Design review of the part built by this model. Coordinates are the model's own, in mm. Give positions to 0.01 mm unless a question says otherwise; leave off trailing zeros. Loops run counter-clockwise (first coordinate to the right, second up) from the corner with the lowest first, then second, coordinate; pieces in that order, holes last. Notation, with made-up numbers: (-4.5, 40) -> (45.5, 40) arc R24 cw to (45.5, 66) -> close; hole circle Ø4 at (73.5, 76). An arc over 180 degrees is marked (long way). Answer in a Markdown table with one row per item. Add a question column.
(1) For line 1 (Y direction, x = -35, z = 2.15); line 2 (X direction, y = -26.5, z = 2.3); line 3 (Y direction, x = -70.5, z = 1.65), list the stretches that pass through material, from the lowest coordinate up.
(2) Consider section A-A on y = -7.5. Write out the cut boundary in (x, z).
(3) For pin 1 (1.5 mm diameter, centred on x = -62, y = -69, fed in from +Z) (3 decimals), flat-tipped, find the tip position at first contact; note if it passes through.
(4) Consider section C-C on y = -75. Write out the cut boundary in (x, z).
(5) Consider section D-D on x = -2.5. Write out the cut boundary in (y, z), then the cut area to 3 significant figures.
(6) Consider section B-B on x = -71.5. Write out the cut boundary in (y, z).
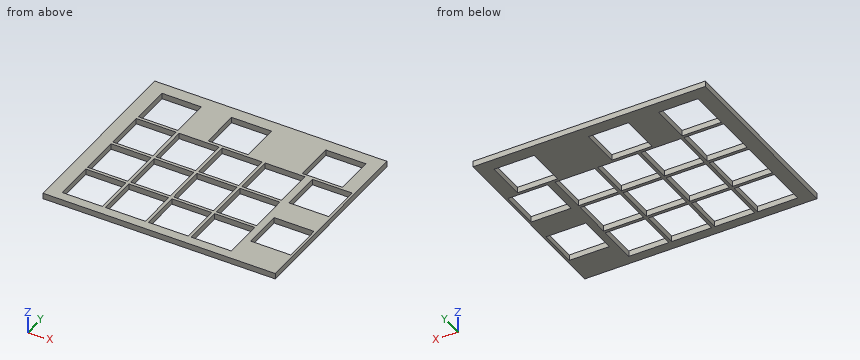
from build123d import *

# Parameters (mm, degrees)
F0_W      = 100
F0_H      = 82
F1_DEPTH  = 2.5
F2_W      = 17.2
F2_H      = 17.2
F3_DEPTH  = 25
F2_W_2    = 17.030713
F4_DEPTH  = 25
F5_W      = 17.2
F5_H      = 17.2
F6_DEPTH  = 25
F7_W      = 17.2
F7_H      = 17.2
F8_DEPTH  = 25
F9_W      = 17.2
F9_H      = 17.2
F10_DEPTH = 25
F11_W     = 17.2
F11_H     = 17.2
F12_DEPTH = 25
F13_W     = 17.2
F13_H     = 17.2
F14_DEPTH = 25
F15_W     = 17.2
F15_H     = 17.2
F16_DEPTH = 25


with BuildPart() as f1:
    # F0 (on Top) → F1 (new body)
    with BuildSketch(Plane.XY):
        with Locations((-39.136762, -41)):
            Rectangle(F0_W, F0_H)
    extrude(amount=F1_DEPTH)

    # F2 (on face) → F3 (cut)
    with BuildSketch(Plane.XY.offset(2.5)):
        with Locations((-74.536762, -69.4)):
            Rectangle(F2_W, F2_H)
    extrude(amount=-F3_DEPTH, mode=Mode.SUBTRACT)

    # F2 (on face) → F4 (cut)
    with BuildSketch(Plane.XY.offset(2.5)):
        with Locations((-74.536762, -69.4)):
            Rectangle(F2_W, F2_H)
        with Locations((-74.536762, -50.9)):
            Rectangle(F2_W, F2_H)
        with Locations((-74.536762, -32.4)):
            Rectangle(F2_W, F2_H)
        with Locations((-74.452118, -13.9)):
            Rectangle(F2_W_2, F2_H)
    extrude(amount=-F4_DEPTH, mode=Mode.SUBTRACT)

    # F5 (on face) → F6 (cut)
    with BuildSketch(Plane.XY.offset(2.5)):
        with Locations((-56.036762, -69.4)):
            Rectangle(F5_W, F5_H)
        with Locations((-37.536762, -69.4)):
            Rectangle(F5_W, F5_H)
        with Locations((-19.036762, -69.4)):
            Rectangle(F5_W, F5_H)
    extrude(amount=-F6_DEPTH, mode=Mode.SUBTRACT)

    # F7 (on face) → F8 (cut)
    with BuildSketch(Plane.XY.offset(2.5)):
        with Locations((-56.036762, -50.9)):
            Rectangle(F7_W, F7_H)
        with Locations((-56.036762, -32.4)):
            Rectangle(F7_W, F7_H)
        with Locations((-37.536762, -50.9)):
            Rectangle(F7_W, F7_H)
        with Locations((-37.536762, -32.4)):
            Rectangle(F7_W, F7_H)
    extrude(amount=-F8_DEPTH, mode=Mode.SUBTRACT)

    # F9 (on face) → F10 (cut)
    with BuildSketch(Plane.XY.offset(2.5)):
        with Locations((-19.036762, -50.9)):
            Rectangle(F9_W, F9_H)
        with Locations((-19.036762, -32.4)):
            Rectangle(F9_W, F9_H)
    extrude(amount=-F10_DEPTH, mode=Mode.SUBTRACT)

    # F11 (on face) → F12 (cut)
    with BuildSketch(Plane.XY.offset(2.5)):
        with Locations((1.263238, -60.4)):
            Rectangle(F11_W, F11_H)
        with Locations((1.263238, -32.4)):
            Rectangle(F11_W, F11_H)
    extrude(amount=-F12_DEPTH, mode=Mode.SUBTRACT)

    # F13 (on face) → F14 (cut)
    with BuildSketch(Plane.XY.offset(2.5)):
        with Locations((-44.336762, -13.9)):
            Rectangle(F13_W, F13_H)
    extrude(amount=-F14_DEPTH, mode=Mode.SUBTRACT)

    # F15 (on face) → F16 (cut)
    with BuildSketch(Plane.XY.offset(2.5)):
        with Locations((-3.736762, -13.9)):
            Rectangle(F15_W, F15_H)
    extrude(amount=-F16_DEPTH, mode=Mode.SUBTRACT)


solid = f1.part
Values follow:
| question | item | result |
|---|---|---|
| 1 | line 1 | -82 to -78, -60.8 to -59.5, -42.3 to -41, -23.8 to 0 |
| 1 | line 2 | -89.14 to -83.14, -65.94 to -64.64, -47.44 to -46.14, -28.94 to -27.64, -10.44 to -7.34, 9.86 to 10.86 |
| 1 | line 3 | -82 to -78, -60.8 to -59.5, -42.3 to -41, -23.8 to -22.5, -5.3 to 0 |
| 2 | outline | (-89.14, 0) -> (-82.97, 0) -> (-82.97, 2.5) -> (-89.14, 2.5) -> close; (-65.94, 0) -> (-52.94, 0) -> (-52.94, 2.5) -> (-65.94, 2.5) -> close; (-35.74, 0) -> (-12.34, 0) -> (-12.34, 2.5) -> (-35.74, 2.5) -> close; (4.86, 0) -> (10.86, 0) -> (10.86, 2.5) -> (4.86, 2.5) -> close |
| 3 | pin 1 | through |
| 4 | outline | (-89.14, 0) -> (-83.14, 0) -> (-83.14, 2.5) -> (-89.14, 2.5) -> close; (-65.94, 0) -> (-64.64, 0) -> (-64.64, 2.5) -> (-65.94, 2.5) -> close; (-47.44, 0) -> (-46.14, 0) -> (-46.14, 2.5) -> (-47.44, 2.5) -> close; (-28.94, 0) -> (-27.64, 0) -> (-27.64, 2.5) -> (-28.94, 2.5) -> close; (-10.44, 0) -> (10.86, 0) -> (10.86, 2.5) -> (-10.44, 2.5) -> close |
| 5 | outline | (-82, 0) -> (-69, 0) -> (-69, 2.5) -> (-82, 2.5) -> close; (-51.8, 0) -> (-41, 0) -> (-41, 2.5) -> (-51.8, 2.5) -> close; (-23.8, 0) -> (-22.5, 0) -> (-22.5, 2.5) -> (-23.8, 2.5) -> close; (-5.3, 0) -> (0, 0) -> (0, 2.5) -> (-5.3, 2.5) -> close |
| 5 | area | 76.0 mm2 |
| 6 | outline | (-82, 0) -> (-78, 0) -> (-78, 2.5) -> (-82, 2.5) -> close; (-60.8, 0) -> (-59.5, 0) -> (-59.5, 2.5) -> (-60.8, 2.5) -> close; (-42.3, 0) -> (-41, 0) -> (-41, 2.5) -> (-42.3, 2.5) -> close; (-23.8, 0) -> (-22.5, 0) -> (-22.5, 2.5) -> (-23.8, 2.5) -> close; (-5.3, 0) -> (0, 0) -> (0, 2.5) -> (-5.3, 2.5) -> close |
